Read the model definition and answer for the solid it produces. Units are mm, in the model's axes. Face numbers are marked on the shaded views. A direction names the side the tool comes from. Give positions to 0.01 mm unless a question says otherwise; leave off trailing zeros. Write each loop counter-clockwise with the first axis right and the second up, starting at its lowest first coordinate (ties: lowest second). Pieces come first, ordered by that corner, then holes.
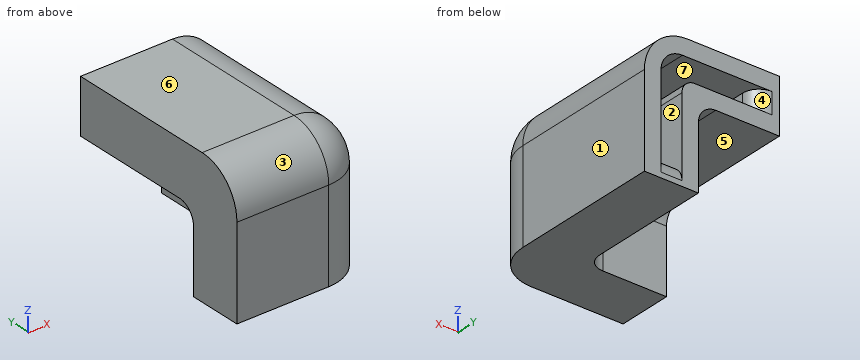
```python
from build123d import *
from OCP.BRepFilletAPI import BRepFilletAPI_MakeFillet

# Parameters (mm, degrees)
BOSS_EXTRUDE1_DEPTH = 18
SKETCH3_W           = 7.5
SKETCH3_H           = 7.5
BOSS_EXTRUDE2_DEPTH = 5
CUT_EXTRUDE1_DEPTH  = 8
FILLET1_R1          = 4
FILLET1_R2          = 1.6
FILLET1_R3          = 1.5


with BuildPart() as part:
    # Sketch1 → Boss-Extrude1 (new body)
    with BuildSketch(Plane(origin=(0, 0, 0), x_dir=(1, 0, 0), z_dir=(0, 1, 0))):
        Polygon((0, 0), (12.5, 0), (12.5, 12.5), (7.5, 12.5), (7.5, 5), (0, 5), align=None)
    extrude(amount=BOSS_EXTRUDE1_DEPTH)

    # Sketch3 → Boss-Extrude2 (add)
    with BuildSketch(Plane.XZ):
        with Locations((3.75, -8.75)):
            Rectangle(SKETCH3_W, SKETCH3_H)
    extrude(amount=-BOSS_EXTRUDE2_DEPTH)

    # Sketch2 → Cut-Extrude1 (cut)
    with BuildSketch(Plane(origin=(0, 18, 0), x_dir=(1, 0, 0), z_dir=(0, 1, 0))):
        with BuildLine():
            Line((9.025, 10.52), (9.025, 4.675))
            ThreePointArc((9.025, 4.675), (8.673528137, 3.826471863), (7.825, 3.475))
            Line((7.825, 3.475), (2.2, 3.475))
            Line((2.2, 3.475), (2.2, 1.525))
            Line((2.2, 1.525), (8.975, 1.525))
            ThreePointArc((8.975, 1.525), (10.389213562, 2.110786438), (10.975, 3.525))
            Line((10.975, 3.525), (10.975, 10.52))
            Line((10.975, 10.52), (9.025, 10.52))
        make_face()
    extrude(amount=-CUT_EXTRUDE1_DEPTH, mode=Mode.SUBTRACT)

    # Fillet1: one fillet with a radius per group of edges: ONE call of the kernel's fillet builder (fillet() takes one radius for all edges)
    fillet1_edges_1 = [part.edges().sort_by_distance(p)[0] for p in [
        (12.5, 9, 0),
        (6.25, 0, 0),
        (12.5, 0, -6.25),
    ]]
    fillet1_edges_2 = [part.edges().sort_by_distance(p)[0] for p in [
        (7.5, 11.5, -5),
        (7.5, 5, -8.75),
        (3.75, 5, -5),
    ]]
    fillet1_edges_3 = [part.edges().sort_by_distance(p)[0] for p in [
        (2.2, 18, -2.5),
        (10, 18, -10.52),
    ]]
    fillet1 = BRepFilletAPI_MakeFillet(part.part.solid().wrapped)
    for e in fillet1_edges_1:
        fillet1.Add(FILLET1_R1, e.wrapped)
    for e in fillet1_edges_2:
        fillet1.Add(FILLET1_R2, e.wrapped)
    for e in fillet1_edges_3:
        fillet1.Add(FILLET1_R3, e.wrapped)
    add(Compound.cast(fillet1.Shape()), mode=Mode.REPLACE)


solid = part.part
```
Item 1: Which of the six approach directions +Z, -Z, +X, -X, +Y, -Y give full straight-line access (tool end or side, diameter ignored) to the marked faces 5, 6 and 7?
Result set:
face 5: -Z, -X, +Y
face 6: +Z, +X, -X, +Y, -Y
face 7: +Y
Item 2: Section A-A (y = 7.5) is taken. Write down the section's boundary in (x, z).
Result set:
outline: (0, -5) - (5.9, -5) arc R1.6 cw to (7.5, -6.6) - (7.5, -12.5) - (12.5, -12.5) - (12.5, -4) arc R4 ccw to (8.5, 0) - (0, 0) - close
Item 3: Find the intervals of material crossed by line 1 along Z through (x, y) = (4.75, 13.25) (3 decimals); line 2 along X through (y, z) = (10.5, -6.5) (3 decimals); line 3 along Y through (x, z) = (3.75, -7.25), in increasing order.
Result set:
line 1: z = -5 to -3.475, -1.525 to 0
line 2: x = 7.497 to 9.025, 10.975 to 12.5
line 3: y = 0 to 5
Item 4: Determine the mould class of the marked faces 1, 2, 3 and 4 for opening direction X: pulls with the +X half, pulls with the -X half, needs draft (parallel to the pull), parting line crosses it, or undercut.
Result set:
face 1: pulls with the +X half
face 2: undercut
face 3: needs draft
face 4: undercut
Item 5: Section B-B (z = -7.75) is taken. Write down the section's boundary in (x, y) (3 decimals), and give its area (3 significant figures).
Result set:
outline: (0, 0) - (8.5, 0) arc R4 ccw to (12.5, 4) - (12.5, 18) - (10.975, 18) - (10.975, 10) - (9.025, 10) - (9.025, 18) - (7.5, 18) - (7.5, 6.6) arc R1.6 cw to (5.9, 5) - (0, 5) - close
area: 109 mm2
Item 6: Section C-C (y = 14.5) is taken. Write down the section's boundary in (x, z) (3 decimals), and give its area (3 significant figures).
Result set:
outline: (0, -5) - (5.9, -5) arc R1.6 cw to (7.5, -6.6) - (7.5, -12.5) - (12.5, -12.5) - (12.5, -4) arc R4 ccw to (8.5, 0) - (0, 0) - close; hole (2.2, -3.475) - (7.825, -3.475) arc R1.2 cw to (9.025, -4.675) - (9.025, -10.52) - (10.975, -10.52) - (10.975, -3.525) arc R2 ccw to (8.975, -1.525) - (2.2, -1.525) - close
area: 66.8 mm2
Item 7: Each of these flat-tipped pins is pushed along its axis until it touches: pin 1 Ø3 at (x, y) = (3.5, 15) entering from -Z; pin 2 Ø1 at (x, y) = (10.5, 13.5) entering from +Z; pin 3 Ø3 at (x, z) = (2, -8.5) entering from +Y. Where does it stop, or does it pass through?
Result set:
pin 1: stops at z = -5
pin 2: stops at z = -0.29
pin 3: stops at y = 5
Item 8: Section D-D (x = 2.5) is taken. Write down the section's boundary in (y, z) (3 decimals).
Result set:
outline: (0, -12.5) - (5, -12.5) - (5, -6.6) arc R1.6 cw to (6.6, -5) - (18, -5) - (18, -3.475) - (10, -3.475) - (10, -1.525) - (18, -1.525) - (18, 0) - (4, 0) arc R4 ccw to (0, -4) - close
